from build123d import *

# Parameters (mm, degrees)
F1_DEPTH = 25.4


with BuildPart() as f1:
    # F0 (on Front) → F1 (new body, symmetric)
    with BuildSketch(Plane.XZ):
        with BuildLine():
            Line((22.225, 9.525), (41.275, 9.525))
            Line((41.275, 9.525), (41.275, 27.0002))
            ThreePointArc((41.275, 27.0002), (45.92468, 38.22552), (57.15, 42.8752))
            Line((57.15, 42.8752), (65.405, 42.8752))
            Line((65.405, 42.8752), (65.405, 61.9252))
            Line((65.405, 61.9252), (57.15, 61.9252))
            add(Edge.make_bspline(
                [(56.590509, 61.920718), (56.776833, 61.922454), (56.963331, 61.923948), (57.15, 61.9252)],
                knots=[111.140328, 111.140328, 111.140328, 111.140328, 111.504536, 111.504536, 111.504536, 111.504536], degree=3))
            ThreePointArc((56.590509, 61.920718), (32.257272, 51.497296), (22.225, 27.0002))
            Line((22.225, 27.0002), (22.225, 9.525))
        make_face()
    extrude(amount=F1_DEPTH, both=True)


solid = f1.part
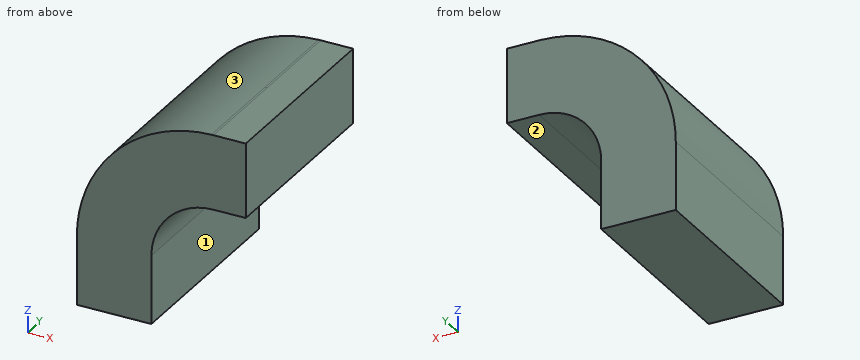
For this review, take the finished solid that the model builds, in its own axes (mm). Face numbers are marked on the shaded views. Give positions to 0.01 mm unless a question says otherwise; leave off trailing zeros. Order: outer loops, then holes, each group sorted by start corner. A loop starts at its lowest first (then second) coordinate and runs counter-clockwise, first axis right, second up. Notation, with made-up numbers: (20.25, 73.25) - (46.25, 73.25) arc R27 cw to (46.25, 100.25) - close; hole circle Ø5 at (20.25, 15.5). An arc over 180 degrees is marked (long way). Answer as a JSON object with one key per item and string values. Group by question number.
Item 1: Wall thickness on line 1 along X through (y, z) = (9, 21.5) (3 decimals); line 2 along Z through (x, y) = (56.5, 9); line 3 along X through (y, z) = (13.5, 56) (3 decimals): over which ranges is each line inside the solid? List them lowest first.
Item 2: Take a section at B-B on x = 26. Give the boundary of the cut face in (y, z) (3 decimals), and give its area (3 significant figures).
Item 3: Draft analysis for pull direction Z (two halves, no side actions). For the marked faces 1, 2 and 3, state which applies: pulls with the +Z half, pulls with the -Z half, needs draft (parallel to the pull), parting line crosses it, or undercut.
Item 4: Take a section at A-A on z = 17. Give the boundary of the cut face in (x, y) (3 decimals), and give its area (3 significant figures).
Item 5: Clearance check with flat-ended pins moving along their axes: pin 1 Ø6.5 at (x, y) = (61, 8) entering from -Z; pin 2 Ø2 at (y, z) = (14, 24.5) entering from +X (3 decimals); pin 3 Ø12 at (y, z) = (-15, 39.5) entering from -X. State where each tip first meets the part, or that it passes through.
Reported:
{
 "1": {"line 1": "22.225 to 41.275", "line 2": "42.86 to 61.92", "line 3": "37.688 to 65.405"},
 "2": {"outline": "(-25.4, 9.525) - (25.4, 9.525) - (25.4, 42.794) - (-25.4, 42.794) - close", "area": "1,690 mm^2"},
 "3": {"face 1": "needs draft", "face 2": "pulls with the -Z half", "face 3": "pulls with the +Z half"},
 "4": {"outline": "(22.225, -25.4) - (41.275, -25.4) - (41.275, 25.4) - (22.225, 25.4) - close", "area": "968 mm^2"},
 "5": {"pin 1": "z = 42.88", "pin 2": "x = 41.275", "pin 3": "x = 22.84"}
}
